Drawing for the job (mm, zero at the part's lowest x, y, z). A direction names the side the tool comes from. Give positions to 0.01 mm unless a question says otherwise; leave off trailing zeros. Write each loop counter-clockwise with the first axis right and the second up, starting at its lowest first coordinate (ties: lowest second). Pieces come first, ordered by that corner, then holes.
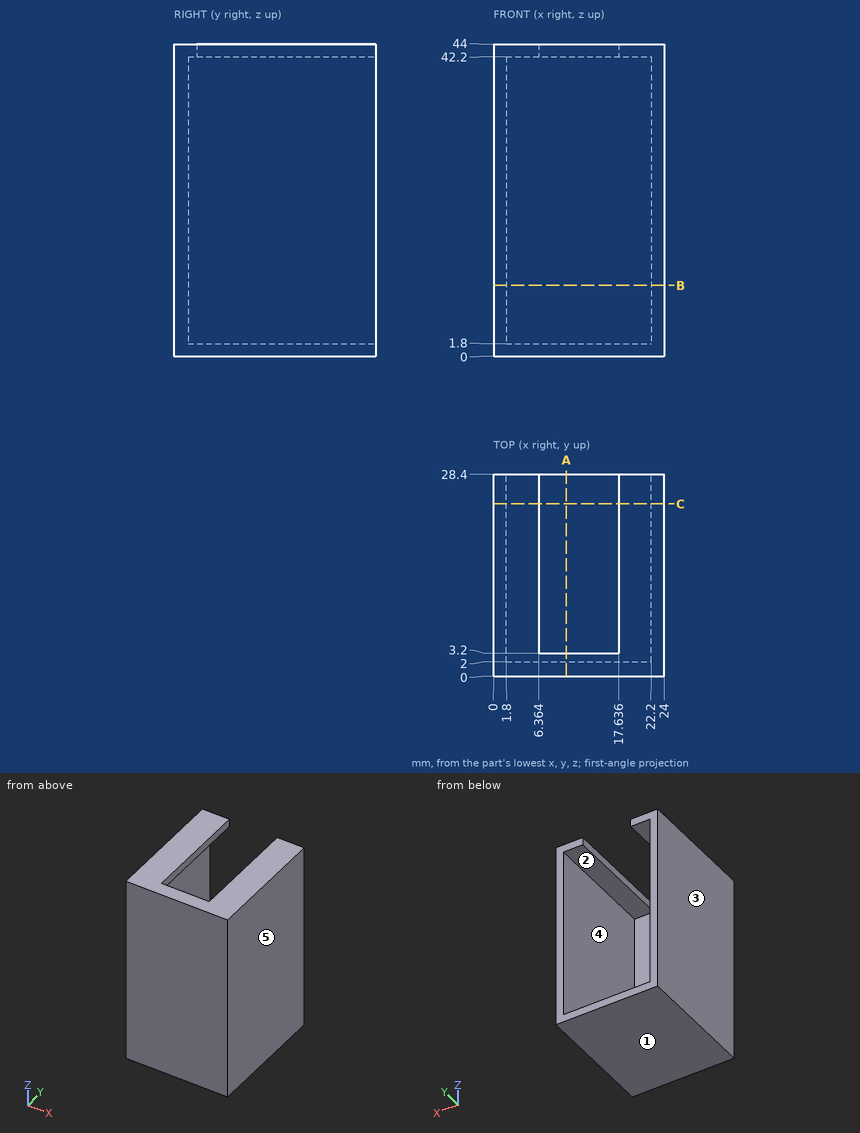
1. Slice it at C-C, the plane y = 24.25. Write the cut outline in (x, z).
Calculated:
outline: (0, 0) - (24, 0) - (24, 44) - (17.64, 44) - (17.64, 42.2) - (22.2, 42.2) - (22.2, 1.8) - (1.8, 1.8) - (1.8, 42.2) - (6.36, 42.2) - (6.36, 44) - (0, 44) - close
2. Slice it at A-A, the plane x = 10.25. Write the cut outline in (y, z).
Calculated:
outline: (0, 0) - (28.4, 0) - (28.4, 1.8) - (2, 1.8) - (2, 42.2) - (3.2, 42.2) - (3.2, 44) - (0, 44) - close
3. Slice it at B-B, the plane z = 10. Write the cut outline in (x, y).
Calculated:
outline: (0, 0) - (24, 0) - (24, 28.4) - (22.2, 28.4) - (22.2, 2) - (1.8, 2) - (1.8, 28.4) - (0, 28.4) - close
4. Probe probe 1 along X at (y, z) = (5.5, 18); probe 2 along Z at (x, y) = (4.5, 6.25); probe 3 along Y at (x, z) = (10, 42). List the from-to ranges inside material, lowest first.
Calculated:
probe 1: x = 0 to 1.8, 22.2 to 24
probe 2: z = 0 to 1.8, 42.2 to 44
probe 3: y = 0 to 2
5. Which spindle directions (+Z, -Z, +X, -X, +Y, -Y) get a long thin tool onto all of the face, cutting with end or side? Do the marked faces 1 and 2. Say none if no direction does.
Calculated:
face 1: -Z, +X, -X, +Y, -Y
face 2: +Y
6. Pin check, flat tips, straight feed: P1, Ø1, axis at x = 8, z = 19.5, coming from the +Y side; P2, Ø5, axis at x = 11, y = 6.5, coming from the +Z side; P3, Ø2, axis at x = 10, z = 43.5, coming from the +Y side. Stop position of each tip, or through.
Calculated:
P1: stops at y = 2
P2: stops at z = 1.8
P3: stops at y = 3.2
7. Pull direction X, two halves, no side cores. Call the marked faces 3, 4 and 5: +X half, -X half, draft (parallel to the pull), parting line (faces both ways), or undercut.
Calculated:
face 3: -X half
face 4: undercut
face 5: +X half
